from build123d import *
from OCP.BRepFilletAPI import BRepFilletAPI_MakeChamfer

# Parameters (mm, degrees)
BOSS_EXTRUDE1_DEPTH = 11.1125
FILLET1_R           = 6.35
FILLET2_R           = 5.715
SKETCH2_R           = 2.365
BOSS_EXTRUDE2_DEPTH = 6.35
BOSS_EXTRUDE3_DEPTH = 2.54
SKETCH4_W           = 1.016
SKETCH4_H           = 8.89
CUT_EXTRUDE2_DEPTH  = 21.94269975
CHAMFER1_SIZE       = 0.79375
CHAMFER1_SIZE2      = 0.458271776
CUT_EXTRUDE3_DEPTH  = 21.94269975


# Some blends are built 0.0001 mm under size
with BuildPart() as part:
    # Sketch1 → Boss-Extrude1 (new body)
    with BuildSketch(Plane.XY):
        with BuildLine():
            Line((3.302, 0), (15.367, 0))
            Line((15.367, 0), (15.367, -6.35))
            Line((15.367, -6.35), (-6.477, -6.35))
            Line((-6.477, -6.35), (-6.477, 0))
            Line((-6.477, 0), (-3.302, 0))
            ThreePointArc((-3.302, 0), (0, -3.302), (3.302, 0))
        make_face()
    extrude(amount=BOSS_EXTRUDE1_DEPTH)

    # Fillet1
    fillet1_edges = [part.edges().sort_by_distance(p)[0] for p in [
        (-6.477, -6.35, 5.55625),
    ]]
    fillet(fillet1_edges, radius=FILLET1_R - 0.0001)  # a hair under: the kernel refuses the full size

    # Fillet2
    # the kernel refuses this fillet: 5.715 mm, written as the material it takes off along each edge
    with BuildSketch(Plane(origin=(15.367, 14.2875, 0), x_dir=(-1, 0, 0), z_dir=(0, -1, 0)), Plane(origin=(15.367, 14.2875, 11.1125), x_dir=(0, 0, -1), z_dir=(0, -1, 0))) as fillet2_piece_1:
        with BuildLine():
            CenterArc((FILLET2_R, -FILLET2_R), FILLET2_R, 90, 90)
            Line((0, -FILLET2_R), (0, 0))
            Line((0, 0), (FILLET2_R, 0))
        make_face()
    extrude(amount=34.925, mode=Mode.SUBTRACT)

    # Sketch2 → Boss-Extrude2 (add)
    with BuildSketch(Plane(origin=(0, 0, 0), x_dir=(1, 0, 0), z_dir=(0, 1, 0))):
        with Locations(Location((9.652, -5.55625, 0), (0, 0, 270))):
            Circle(SKETCH2_R)
    extrude(amount=BOSS_EXTRUDE2_DEPTH)

    # Sketch3 → Boss-Extrude3 (add)
    with BuildSketch(Plane(origin=(0, 6.35, 0), x_dir=(1, 0, 0), z_dir=(0, 1, 0))):
        with BuildLine():
            Line((8.25654631, -7.92125), (11.04745369, -7.92125))
            ThreePointArc((11.04745369, -7.92125), (12.398, -5.55625), (11.04745369, -3.19125))
            Line((11.04745369, -3.19125), (8.25654631, -3.19125))
            ThreePointArc((8.25654631, -3.19125), (6.906, -5.55625), (8.25654631, -7.92125))
        make_face()
    extrude(amount=BOSS_EXTRUDE3_DEPTH)

    # Sketch4 → Cut-Extrude2 (cut, through all)
    with BuildSketch(Plane.XY):
        with Locations((9.652, 4.445)):
            Rectangle(SKETCH4_W, SKETCH4_H)
    extrude(amount=CUT_EXTRUDE2_DEPTH, mode=Mode.SUBTRACT)

    # Chamfer1: one chamfer whose edges measure the first distance from different faces: ONE call of the kernel's chamfer builder (chamfer() names one face for all edges)
    chamfer1_edges_1 = [part.edges().sort_by_distance(p)[0] for p in [
        (6.906, 8.89, 5.55625),
    ]]
    chamfer1_side_1 = [part.faces().sort_by_distance(p)[0] for p in [
        (6.906, 7.62, 5.55625),
    ]]
    chamfer1_edges_2 = [part.edges().sort_by_distance(p)[0] for p in [
        (12.398, 8.89, 5.55625),
    ]]
    chamfer1_side_2 = [part.faces().sort_by_distance(p)[0] for p in [
        (12.398, 7.62, 5.55625),
    ]]
    chamfer1 = BRepFilletAPI_MakeChamfer(part.part.solid().wrapped)
    for e in chamfer1_edges_1:
        chamfer1.Add(CHAMFER1_SIZE, CHAMFER1_SIZE2, e.wrapped, chamfer1_side_1[0].wrapped)  # the first distance lies on this face
    for e in chamfer1_edges_2:
        chamfer1.Add(CHAMFER1_SIZE, CHAMFER1_SIZE2, e.wrapped, chamfer1_side_2[0].wrapped)  # the first distance lies on this face
    add(Compound.cast(chamfer1.Shape()), mode=Mode.REPLACE)

    # Sketch5 → Cut-Extrude3 (cut, through all)
    with BuildSketch(Plane(origin=(0, 0, 0), x_dir=(1, 0, 0), z_dir=(0, 1, 0))):
        with BuildLine():
            Line((9.652, 0), (-6.477, 0))
            Line((-6.477, 0), (-6.477, -11.1125))
            Line((-6.477, -11.1125), (9.652, -11.1125))
            ThreePointArc((9.652, -11.1125), (4.09575, -5.55625), (9.652, 0))
        make_face()
    extrude(amount=-CUT_EXTRUDE3_DEPTH, mode=Mode.SUBTRACT)


solid = part.part
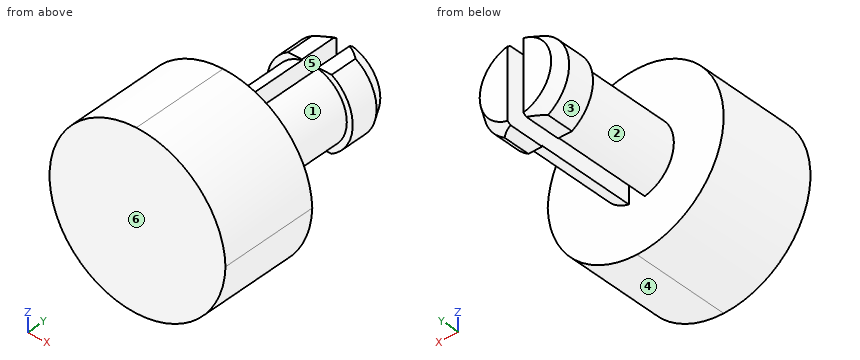
Design review of the part built by this model. Coordinates are the model's own, in mm. Face numbers are marked on the shaded views. A direction names the side the tool comes from. Coordinates: 2 decimals unless noted, no trailing zeros. Loops run counter-clockwise (first coordinate to the right, second up) from the corner with the lowest first, then second, coordinate; pieces in that order, holes last. Notation, with made-up numbers: M 25.25,55.25 L 39.25,55.25 A19 ccw 39.25,87.25 Z; hole C -37,50 d6. An arc over 180 degrees is marked long. Use one line per item in the form item = value.
(1) Draft analysis for pull direction X (two halves, no side actions). For the marked faces 4, 5 and 6, state which applies: pulls with the +X half, pulls with the -X half, needs draft (parallel to the pull), parting line crosses it, or undercut.
Return value:
face_4 = pulls with the +X half
face_5 = undercut
face_6 = needs draft
(2) Consider section D-D (x = 13.75). Write out the cut boundary in (y, z).
Return value:
outline = M -6.35,1.73 L 0,1.73 L 0,9.38 L -6.35,9.38 Z
(3) Consider section A-A (y = 7.75). Write out the cut boundary in (x, z), and give its area (3 significant figures).
Return value:
outline = M 8.26,3.19 L 9.14,3.19 L 9.14,7.92 L 8.26,7.92 A2.75 ccw Z; M 10.16,3.19 L 11.05,3.19 A2.75 ccw 11.05,7.92 L 10.16,7.92 Z
area = 17.4 mm2
(4) Consider section C-C (z = 9.75). Write out the cut boundary in (x, y), and give its area (3 significant figures).
Return value:
outline = M 6.01,-6.35 L 13.36,-6.35 L 13.36,0 L 6.01,0 Z
area = 46.7 mm2
(5) Clearance check with flat-ended pins moving along their axes: P1, Ø5, axis at y = 4, z = 5, coming from the -X side; P2, Ø1.4, axis at y = 3.5, z = 4.5, coming from the +X side; P3, Ø1, axis at x = 10.5, y = 7.5, coming from the +Z side. State where each tip first meets the part, or that it passes through.
Return value:
P1 = 6.91
P2 = 11.99
P3 = 7.92
(6) For the marked faces 1, 2 and 3, list the 3-axis set-ups (+Z, -Z, +X, -X, +Y, -Y) from which the entire face can be reached by the end or side of a thin tool; tool diameter is ignored.
Return value:
face_1 = +X
face_2 = -X
face_3 = -X, +Y
(7) For line 1 along Y through (x, z) = (11.25, 1.5); line 2 along X through (y, z) = (2.25, 4); line 3 along Z through (x, y) = (8.25, 7.75), list the stretches that pass through material, from the lowest coordinate up. Write a range as from..to.
Return value:
line_1 = -6.35..0
line_2 = 7.87..9.14, 10.16..11.43
line_3 = 3.2..7.92
